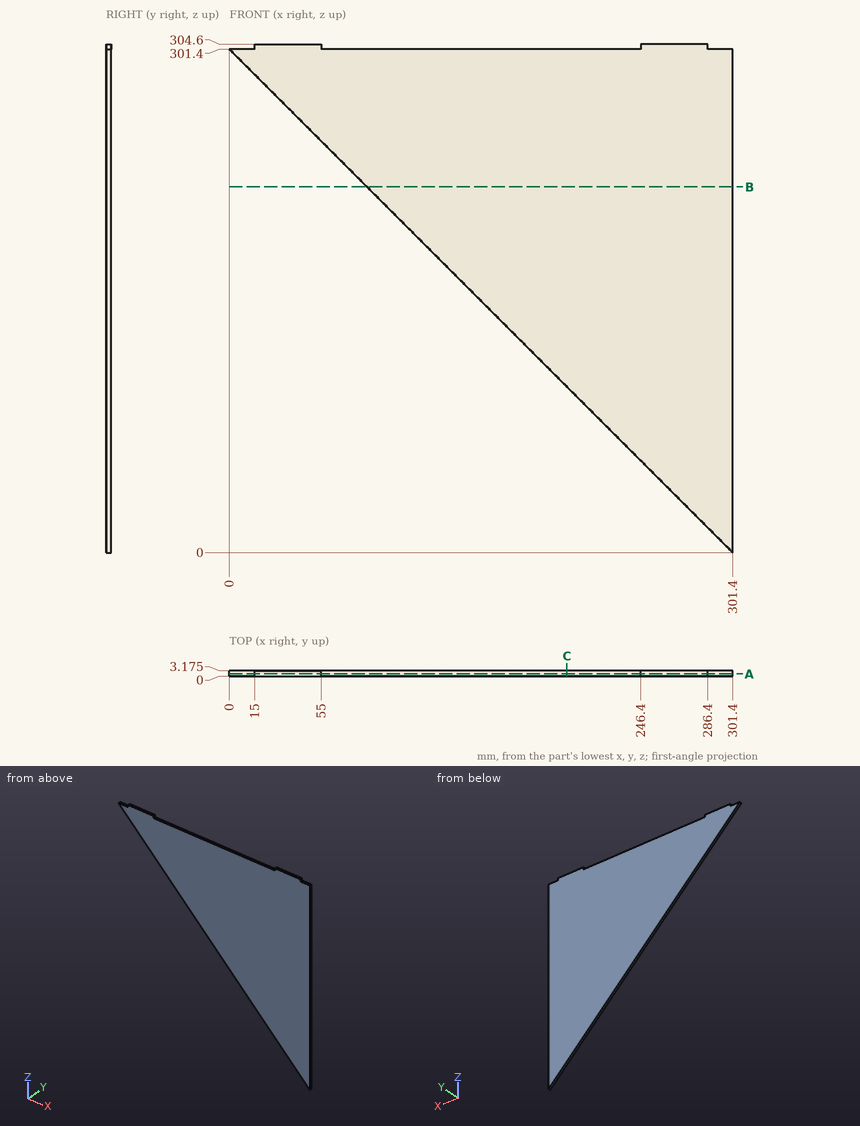
Geometry check sheet. Reference: drawing and pictorial views, mm from the part's lowest x, y, z. Round coordinates to 2 decimals unless told otherwise and drop trailing zeros. Loops run counter-clockwise (first coordinate to the right, second up) from the corner with the lowest first, then second, coordinate; pieces in that order, holes last. Notation, with made-up numbers: (74, 86.25) - (91, 86.25) arc R29 ccw to (91, 110.25) - close; hole circle Ø8 at (78.25, -28.75). An arc over 180 degrees is marked (long way). Answer in a Markdown table with one row per item. Add a question column.
Q1. Section check B-B on z = 219. Enter the section's corners in (x, y) (3 decimals).
Q2. Section check A-A on y = 1.2. Enter the section's corners in (x, z).
Q3. Material ranges on line 1 (Z direction, x = 39.5, y = 1.75); line 2 (Z direction, x = 30, y = 0.85); line 3 (X direction, y = 1.9, z = 290), recorded low to high.
Q4. Section check C-C on x = 202. Enter the section's corners in (y, z) (3 decimals).
Q5. Gauge pin test, flat ends, axial feed: pin 1 (1 mm diameter, centred on y = 1, z = 268, fed in from -X); pin 2 (1.6 mm diameter, centred on y = 2, z = 302.5, fed in from +X); pin 3 (1.6 mm diameter, centred on x = 10, y = 1.5, fed in from +Z). Record the tip position at first contact, or that the pin passes through.
Found:
| question | item | result |
|---|---|---|
| 1 | outline | (82.4, 0) - (301.4, 0) - (301.4, 3.175) - (82.4, 3.175) - close |
| 2 | outline | (0, 301.4) - (301.4, 0) - (301.4, 301.4) - (286.4, 301.4) - (286.4, 304.6) - (246.4, 304.6) - (246.4, 301.4) - (55, 301.4) - (55, 304.6) - (15, 304.6) - (15, 301.4) - close |
| 3 | line 1 | z = 261.9 to 304.6 |
| 3 | line 2 | z = 271.4 to 304.6 |
| 3 | line 3 | x = 11.4 to 301.4 |
| 4 | outline | (0, 99.4) - (3.175, 99.4) - (3.175, 301.4) - (0, 301.4) - close |
| 5 | pin 1 | stops at x = 32.9 |
| 5 | pin 2 | stops at x = 286.4 |
| 5 | pin 3 | stops at z = 301.4 |
